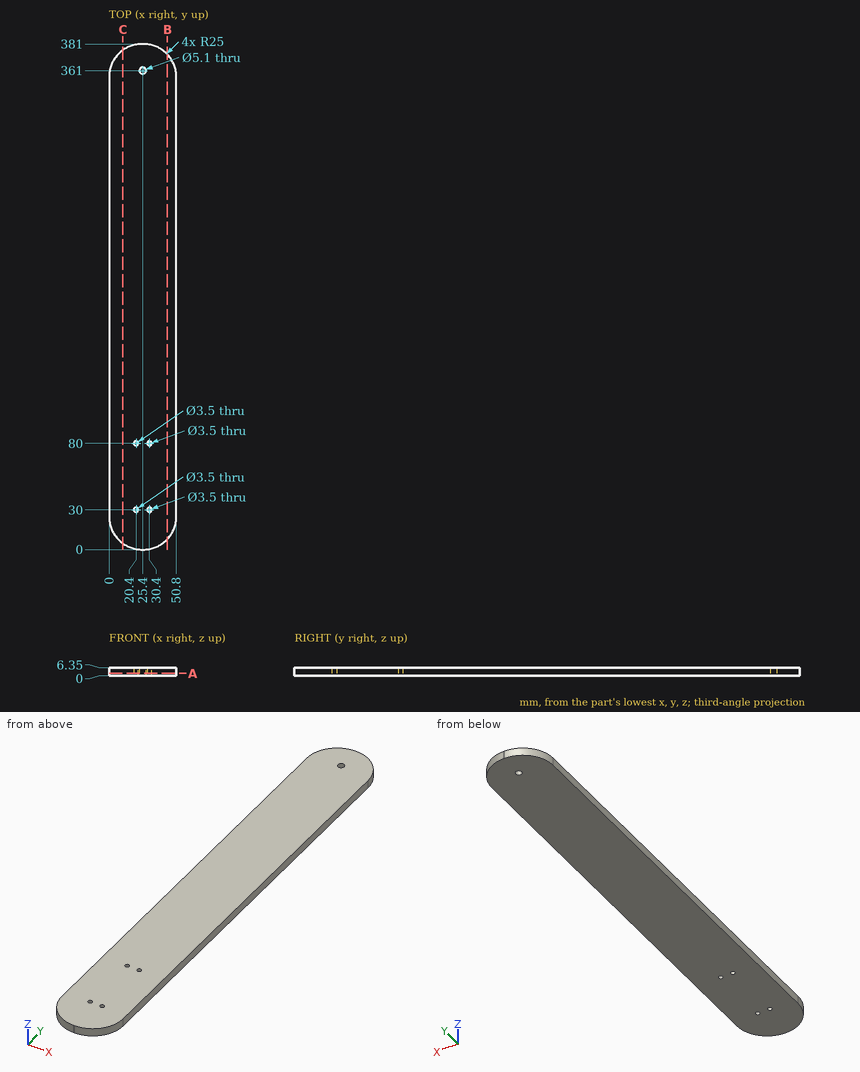
Input: dimensioned drawing with shaded views. Units: mm. Origin: part minimum x, y, z. Give positions to 0.01 mm unless a question says otherwise; leave off trailing zeros. Write each loop counter-clockwise with the first axis right and the second up, starting at its lowest first coordinate (ties: lowest second). Pieces come first, ordered by that corner, then holes.
1. Material intervals for line 1 along Y through (x, z) = (30, 3.75); line 2 along Y through (x, z) = (25.4, 3.75); line 3 along X through (y, z) = (356.5, 2.75) (3 decimals), sorted ascending.
2. Section query C-C (x = 10.5). Return the cut outline in (y, z).
3. Section query A-A (z = 2). Return the cut outline in (x, y), then the cut area to 3 significant figures.
4. First-contact query: pin 1 (2 mm diameter, centred on x = 30.5, z = 5.5, fed in from +Y). Flat tip, straight axial feed; report the tip coordinate or a pass-through.
5. Section query B-B (x = 44). Return the cut outline in (y, z).
Output values:
1. line 1: y = 0.36 to 28.3, 31.7 to 78.3, 81.7 to 380.64
1. line 2: y = 0 to 358.45, 363.55 to 381
1. line 3: x = 0.005 to 50.795
2. outline: (4.63, 0) - (376.37, 0) - (376.37, 6.35) - (4.63, 6.35) - close
3. outline: (0, 25) arc R25 ccw to (25, 0) - (25.8, 0) arc R25 ccw to (50.8, 25) - (50.8, 356) arc R25 ccw to (25.8, 381) - (25, 381) arc R25 ccw to (0, 356) - close; hole circle Ø3.5 at (20.4, 30); hole circle Ø3.5 at (20.4, 80); hole circle Ø5.1 at (25.4, 361); hole circle Ø3.5 at (30.4, 30); hole circle Ø3.5 at (30.4, 80)
3. area: 18,800 mm2
4. pin 1: stops at y = 380.72
5. outline: (7.86, 0) - (373.14, 0) - (373.14, 6.35) - (7.86, 6.35) - close
